Geometry: final body of the model. Coordinates: model frame, mm. Face numbers are marked on the shaded views. A direction names the side the tool comes from. Give positions to 0.01 mm unless a question says otherwise; leave off trailing zeros. Order: outer loops, then holes, each group sorted by start corner. A loop starts at its lowest first (then second) coordinate and runs counter-clockwise, first axis right, second up. Notation, with made-up numbers: (-10, -15) -> (5, -15) arc R23 cw to (5, 19) -> close; hole circle Ø8 at (77.5, 34.25). An arc over 180 degrees is marked (long way). Write item = value, one per line.
```python
from build123d import *

# Parameters (mm, degrees)
SKETCH1_W           = 22.86
SKETCH1_H           = 12.192
BOSS_EXTRUDE1_DEPTH = 22.352
BOSS_EXTRUDE2_DEPTH = 4.318
BOSS_EXTRUDE3_START = -15.748
BOSS_EXTRUDE3_DEPTH = 2.54
SKETCH4_R           = 2.413
SKETCH4_R_2         = 1.016
BOSS_EXTRUDE4_DEPTH = 3.048


with BuildPart() as part:
    # Sketch1 → Boss-Extrude1 (new body)
    with BuildSketch(Plane(origin=(0, 0, 0), x_dir=(1, 0, 0), z_dir=(0, 1, 0))):
        Rectangle(SKETCH1_W, SKETCH1_H)
    extrude(amount=BOSS_EXTRUDE1_DEPTH)

    # Sketch2 → Boss-Extrude2 (add)
    with BuildSketch(Plane(origin=(0, 22.352, 0), x_dir=(1, 0, 0), z_dir=(0, 1, 0))):
        with BuildLine():
            Line((0.762, 3.475776023), (-0.325986717, 3.475776023))
            ThreePointArc((-0.325986717, 3.475776023), (-11.43, 0), (-0.325986717, -3.475776023))
            Line((-0.325986717, -3.475776023), (0.762, -3.475776023))
            ThreePointArc((0.762, -3.475776023), (4.237776023, 0), (0.762, 3.475776023))
        make_face()
    extrude(amount=BOSS_EXTRUDE2_DEPTH)

    # Sketch3 → Boss-Extrude3 (add)
    with BuildSketch(Plane.XZ.offset(BOSS_EXTRUDE3_START)):
        with BuildLine():
            Line((-16.129, -6.096), (16.129, -6.096))
            Line((16.129, -6.096), (16.129, -0.613485199))
            Line((16.129, -0.613485199), (15.199445863, -0.613485199))
            ThreePointArc((15.199445863, -0.613485199), (12.827148451, 0.036418828), (15.218207768, 0.613485199))
            Line((15.218207768, 0.613485199), (16.129, 0.613485199))
            Line((16.129, 0.613485199), (16.129, 6.096))
            Line((16.129, 6.096), (-16.129, 6.096))
            Line((-16.129, 6.096), (-16.129, 0.613485199))
            Line((-16.129, 0.613485199), (-15.218207768, 0.613485199))
            ThreePointArc((-15.218207768, 0.613485199), (-12.827148451, 0.036418828), (-15.199445863, -0.613485199))
            Line((-15.199445863, -0.613485199), (-16.129, -0.613485199))
            Line((-16.129, -0.613485199), (-16.129, -6.096))
        make_face()
    extrude(amount=-BOSS_EXTRUDE3_DEPTH)

    # Sketch4 → Boss-Extrude4 (add)
    with BuildSketch(Plane(origin=(0, 26.67, 0), x_dir=(1, 0, 0), z_dir=(0, 1, 0))):
        with Locations((-5.334, 0)):
            Circle(SKETCH4_R)
        with Locations((-5.334, 0)):
            Circle(SKETCH4_R_2, mode=Mode.SUBTRACT)
    extrude(amount=BOSS_EXTRUDE4_DEPTH)


solid = part.part
```
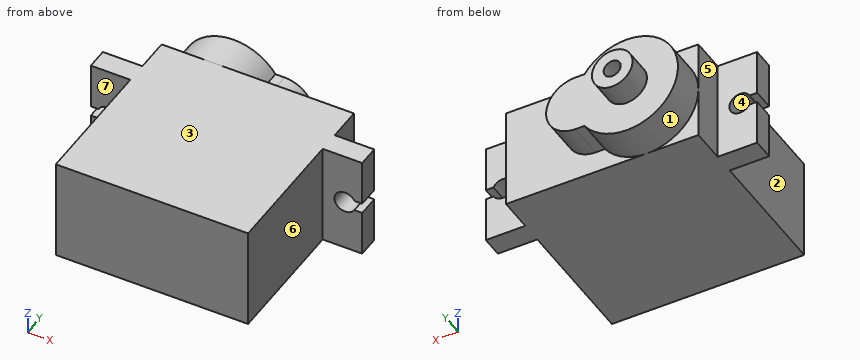
1) Reachability of the marked faces 5, 6 and 7 from +Z, -Z, +X, -X, +Y, -Y: full face, straight path, thin tool, end or side. Return the list, or none.
Check sheet entries:
face_5 = +Z, -Z, -X, +Y
face_6 = +Z, -Z, +X, -Y
face_7 = +Z, -Z, -X, -Y
2) Section query C-C (z = 5.5). Output: boundary loops of the cut face in (x, y), plus the area to 3 significant figures.
Check sheet entries:
outline = (-16.13, 15.75) -> (-11.43, 15.75) -> (-11.43, 0) -> (11.43, 0) -> (11.43, 15.75) -> (16.13, 15.75) -> (16.13, 18.29) -> (11.43, 18.29) -> (11.43, 22.35) -> (-2.71, 22.35) -> (-2.71, 26.67) -> (-7.96, 26.67) -> (-7.96, 22.35) -> (-11.43, 22.35) -> (-11.43, 18.29) -> (-16.13, 18.29) -> close
area = 558 mm²
3) Section query A-A (x = 9). Output: boundary loops of the cut face in (y, z), plus the area to 3 significant figures.
Check sheet entries:
outline = (0, -6.1) -> (22.35, -6.1) -> (22.35, 6.1) -> (0, 6.1) -> close
area = 273 mm²
4) Mould query, pull axis Z, two halves, no side actions, for the marked faces 1, 2, 3 and 4. Classes: +Z half, -Z half, draft (parallel to the pull), parting line (faces both ways), or undercut.
Check sheet entries:
face_1 = parting line
face_2 = draft
face_3 = +Z half
face_4 = undercut
5) First-contact query: P1, Ø4, axis at x = 13.5, z = -0.5, coming from the +Y side; P2, Ø1.8, axis at x = -10, z = 2, coming from the +Y side; P3, Ø4, axis at y = 7.5, z = 1.5, coming from the +X side. Flat tips, straight axial feed; report the tip coordinate or a pass-through.
Check sheet entries:
P1 = 18.29
P2 = 26.67
P3 = 11.43
6) Section query B-B (y = 26). Output: boundary loops of the cut face in (x, z).
Check sheet entries:
outline = (-0.33, -3.48) -> (0.76, -3.48) arc R3.48 ccw to (0.76, 3.48) -> (-0.33, 3.48) arc R6.1 ccw (long way) to start
7) Line query: line 1 (X direction, y = 17.5, z = 0.75); line 2 (X direction, y = 20.75, z = 2.5); line 3 (Y direction, x = -5.5, z = 3.5). Output: solid intervals per line, ascending. Write a range as from..to.
Check sheet entries:
line_1 = -16.13..-15.13, -13.06..13.06, 15.13..16.13
line_2 = -11.43..11.43
line_3 = 0..26.67
